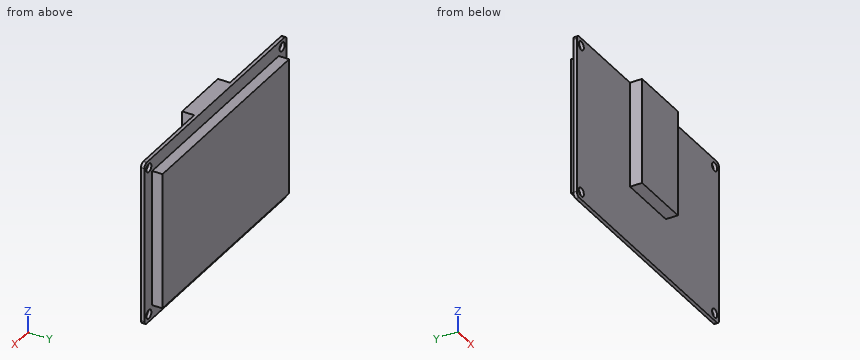
from build123d import *

# Parameters (mm, degrees)
SKETCH1_W           = 70
SKETCH1_H           = 48
SKETCH1_R           = 1.25
BOSS_EXTRUDE1_DEPTH = 1
SKETCH2_W           = 62.3
SKETCH2_H           = 40
BOSS_EXTRUDE2_DEPTH = 3
SKETCH4_W           = 17.6
SKETCH4_H           = 31
BOSS_EXTRUDE3_DEPTH = 3.5
FILLET1_R           = 1.2


with BuildPart() as part:
    # Sketch1 → Boss-Extrude1 (new body)
    with BuildSketch(Plane(origin=(0, 0, 0), x_dir=(1, 0, 0), z_dir=(0, 1, 0))):
        Rectangle(SKETCH1_W, SKETCH1_H)
        with Locations(Location((-32.8, 21.8, 0), (0, 0, 270))):
            Circle(SKETCH1_R, mode=Mode.SUBTRACT)
        with Locations(Location((-32.8, -21.8, 0), (0, 0, 90))):
            Circle(SKETCH1_R, mode=Mode.SUBTRACT)
        with Locations(Location((32.8, -21.8, 0), (0, 0, 270))):
            Circle(SKETCH1_R, mode=Mode.SUBTRACT)
        with Locations(Location((32.8, 21.8, 0), (0, 0, 90))):
            Circle(SKETCH1_R, mode=Mode.SUBTRACT)
    extrude(amount=BOSS_EXTRUDE1_DEPTH)

    # Sketch2 → Boss-Extrude2 (add)
    with BuildSketch(Plane(origin=(0, 1, 0), x_dir=(1, 0, 0), z_dir=(0, 1, 0))):
        Rectangle(SKETCH2_W, SKETCH2_H)
    extrude(amount=BOSS_EXTRUDE2_DEPTH)

    # Sketch4 → Boss-Extrude3 (add)
    with BuildSketch(Plane.XZ):
        with Locations((0, 8.5)):
            Rectangle(SKETCH4_W, SKETCH4_H)
    extrude(amount=BOSS_EXTRUDE3_DEPTH)

    # Fillet1
    fillet1_edges = [part.edges().sort_by_distance(p)[0] for p in [
        (35, 0.5, 24),
        (-35, 0.5, 24),
        (-35, 0.5, -24),
        (35, 0.5, -24),
    ]]
    fillet(fillet1_edges, radius=FILLET1_R)


solid = part.part
Could you check a few things on this model? Use its own coordinates, in mm. Give positions to 0.01 mm unless a question says otherwise; leave off trailing zeros. Loops run counter-clockwise (first coordinate to the right, second up) from the corner with the lowest first, then second, coordinate; pieces in that order, holes last. Notation, with made-up numbers: M 62.25,25 L 69.25,25 A15 cw 69.25,38 Z; hole C 76.25,18.5 d5. An arc over 180 degrees is marked long. Answer as a JSON object with one key per item and string values.
Q1. Suppose I cut it at D-D, the plane z = -1. List the corners of the cut face in (x, y) for me, plus the area to 4 significant figures.
Values found:
{"outline": "M -35,0 L -8.8,0 L -8.8,-3.5 L 8.8,-3.5 L 8.8,0 L 35,0 L 35,1 L 31.15,1 L 31.15,4 L -31.15,4 L -31.15,1 L -35,1 Z", "area": "318.5 mm²"}
Q2. Suppose I cut it at B-B, the plane x = 22.5. List the corners of the cut face in (y, z) for me, plus the area to 3 significant figures.
Values found:
{"outline": "M 0,-24 L 1,-24 L 1,-20 L 4,-20 L 4,20 L 1,20 L 1,24 L 0,24 Z", "area": "168 mm²"}
Q3. If I drill on probe 1 along X at (y, z) = (0.4, -21.8); probe 2 along Y at (x, z) = (-16.5, 15.5); probe 3 along X at (y, z) = (-2.75, 4), over which ranges is the centre line in solid material (lowest first)? Write a range as [from, to].
Values found:
{"probe 1": "x = [-35, -34.05], [-31.55, 31.55], [34.05, 35]", "probe 2": "y = [0, 4]", "probe 3": "x = [-8.8, 8.8]"}
Q4. For P1, Ø0.9, axis at x = -12.5, y = 2, coming from the -Z side; P2, Ø4, axis at x = -32.8, z = -21.8, coming from the +Y side; P3, Ø1.5, axis at x = 6.5, y = 3, coming from the +Z side, each with a flat end and sliding along its axis, tell me the tip position at first contact or that it passes through.
Values found:
{"P1": "stops at z = -20", "P2": "stops at y = 1", "P3": "stops at z = 20"}
Q5. Suppose I cut it at A-A, the plane z = 21.8. List the corners of the cut face in (x, y) for me.
Values found:
{"outline": "M -35,0 L -34.05,0 L -34.05,1 L -35,1 Z; M -31.55,0 L -8.8,0 L -8.8,-3.5 L 8.8,-3.5 L 8.8,0 L 31.55,0 L 31.55,1 L -31.55,1 Z; M 34.05,0 L 35,0 L 35,1 L 34.05,1 Z"}
Q6. Suppose I cut it at C-C, the plane x = 32.8. List the corners of the cut face in (y, z) for me, plus the area to 3 significant figures.
Values found:
{"outline": "M 0,-24 L 1,-24 L 1,-23.05 L 0,-23.05 Z; M 0,-20.55 L 1,-20.55 L 1,20.55 L 0,20.55 Z; M 0,23.05 L 1,23.05 L 1,24 L 0,24 Z", "area": "43.0 mm²"}
